The listing builds one solid part. Answer for the finished solid, in the listing's coordinates (mm). Face numbers are marked on the shaded views. A direction names the side the tool comes from. Coordinates: 2 decimals unless noted, no trailing zeros. Loops run counter-clockwise (first coordinate to the right, second up) from the corner with the lowest first, then second, coordinate; pieces in that order, holes last. Notation, with made-up numbers: (84, 29) - (138, 29) arc R17 ccw to (138, 57) - close; hole circle Ø7 at (67, 48). An arc over 180 degrees is marked (long way). Return JSON: item names as keys, results as strings. Group by question number.
1. Find the intervals of material crossed by line 1 along Y through (x, z) = (157.5, 240.5); line 2 along Z through (x, y) = (274.5, 982); line 3 along Z through (x, y) = (159, 373.5), in increasing order.
2. This flat-tipped pin is pushed along its axis until it touches: P1, Ø2, axis at x = 244.5, z = 167, coming from the -Y side. Where does it stop, or does it pass through?
3. Section C-C (y = 583.5) is taken. Write down the section's boundary in (x, z), and give its area (3 significant figures).
4. Which of the six approach directions +Z, -Z, +X, -X, +Y, -Y give full straight-line access (tool end or side, diameter ignored) to the marked faces 1 and 2?
5. Section B-B (z = 215) is taken. Write down the section's boundary in (x, y), and give its area (3 significant figures).
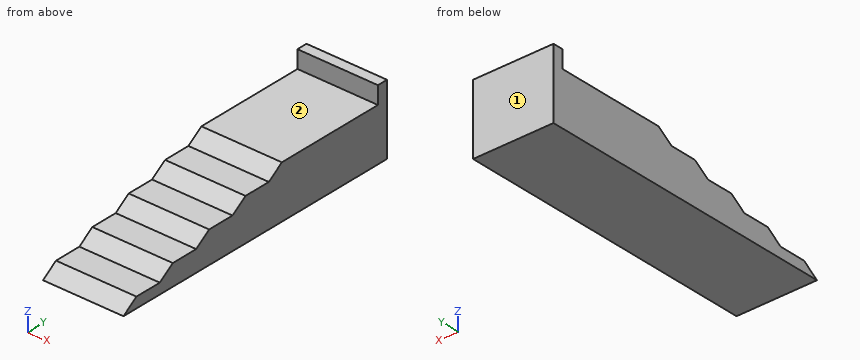
```python
from build123d import *

# Parameters (mm, degrees)
F0_W        = 1066.8
F0_H        = 38.1
F1_DEPTH    = 292.1
F2_W        = 914.4
F2_H        = 38.1
F3_DEPTH    = 292.1
F4_W        = 762
F4_H        = 38.1
F5_DEPTH    = 292.1
F6_W        = 609.6
F6_H        = 38.1
F7_DEPTH    = 292.1
F8_W        = 457.2
F8_H        = 38.1
F9_DEPTH    = 292.1
F10_SIZE2   = 54.412429
F10_SIZE    = 38.09999
F10_2_SIZE2 = 54.412429
F10_2_SIZE  = 38.09999
F10_3_SIZE2 = 54.412429
F10_3_SIZE  = 38.09999
F10_4_SIZE2 = 54.412429
F10_4_SIZE  = 38.09999
F10_5_SIZE2 = 54.412429
F10_5_SIZE  = 38.09999
F11_W       = 292.1000000001
F11_H       = 38.1
F12_DEPTH   = 254


# Not quite as in the source:
# - a fillet or chamfer is up to 0.001 mm smaller than in the source, because OpenCascade refuses the exact size


with BuildPart() as f1:
    # F0 (on Right) → F1 (new body)
    with BuildSketch(Plane.YZ):
        with Locations((533.4, 19.05)):
            Rectangle(F0_W, F0_H)
    extrude(amount=F1_DEPTH)

    # F2 (on Right) → F3 (join, through all)
    with BuildSketch(Plane.YZ):
        with Locations((609.6, 57.15)):
            Rectangle(F2_W, F2_H)
    extrude(amount=F3_DEPTH)

    # F4 (on Right) → F5 (join, through all)
    with BuildSketch(Plane.YZ):
        with Locations((685.8, 95.25)):
            Rectangle(F4_W, F4_H)
    extrude(amount=F5_DEPTH)

    # F6 (on Right) → F7 (join, through all)
    with BuildSketch(Plane.YZ):
        with Locations((762, 133.35)):
            Rectangle(F6_W, F6_H)
    extrude(amount=F7_DEPTH)

    # F8 (on Right) → F9 (join, through all)
    with BuildSketch(Plane.YZ):
        with Locations((838.2, 171.45)):
            Rectangle(F8_W, F8_H)
    extrude(amount=F9_DEPTH)

    # F10 (size 38.1 and 54.4124390569 in the source; OpenCascade refuses exactly that, so slightly less here)
    f10_edges = [f1.edges().sort_by_distance(p)[0] for p in [
        (146.05, 0, 38.1),
    ]]
    f10_side = f1.faces().sort_by_distance((146.05, 0, 19.05))[0]
    chamfer(f10_edges, length=F10_SIZE, length2=F10_SIZE2, reference=f10_side)

    # F10#2 (size 38.1 and 54.4124390569 in the source; OpenCascade refuses exactly that, so slightly less here)
    f10_2_edges = [f1.edges().sort_by_distance(p)[0] for p in [
        (146.05, 152.4, 76.2),
    ]]
    f10_2_side = f1.faces().sort_by_distance((146.05, 152.4, 57.15))[0]
    chamfer(f10_2_edges, length=F10_2_SIZE, length2=F10_2_SIZE2, reference=f10_2_side)

    # F10#3 (size 38.1 and 54.4124390569 in the source; OpenCascade refuses exactly that, so slightly less here)
    f10_3_edges = [f1.edges().sort_by_distance(p)[0] for p in [
        (146.05, 304.8, 114.3),
    ]]
    f10_3_side = f1.faces().sort_by_distance((146.05, 304.8, 95.25))[0]
    chamfer(f10_3_edges, length=F10_3_SIZE, length2=F10_3_SIZE2, reference=f10_3_side)

    # F10#4 (size 38.1 and 54.4124390569 in the source; OpenCascade refuses exactly that, so slightly less here)
    f10_4_edges = [f1.edges().sort_by_distance(p)[0] for p in [
        (146.05, 457.2, 152.4),
    ]]
    f10_4_side = f1.faces().sort_by_distance((146.05, 457.2, 133.35))[0]
    chamfer(f10_4_edges, length=F10_4_SIZE, length2=F10_4_SIZE2, reference=f10_4_side)

    # F10#5 (size 38.1 and 54.4124390569 in the source; OpenCascade refuses exactly that, so slightly less here)
    f10_5_edges = [f1.edges().sort_by_distance(p)[0] for p in [
        (146.05, 609.6, 190.5),
    ]]
    f10_5_side = f1.faces().sort_by_distance((146.05, 609.6, 171.45))[0]
    chamfer(f10_5_edges, length=F10_5_SIZE, length2=F10_5_SIZE2, reference=f10_5_side)

    # F11 (on Top) → F12 (join)
    with BuildSketch(Plane.XY):
        with Locations((146.0500000001, 1085.85)):
            Rectangle(F11_W, F11_H)
    extrude(amount=F12_DEPTH)


solid = f1.part
```
The answers:
{
 "1": {"line 1": "y = 1066.8 to 1104.9", "line 2": "z = 0 to 190.5", "line 3": "z = 0 to 114.3"},
 "2": {"P1": "stops at y = 629.02"},
 "3": {"outline": "(0, 0) - (292.1, 0) - (292.1, 152.4) - (0, 152.4) - close", "area": "44,500 mm2"},
 "4": {"face 1": "+Z, -Z, +X, -X, +Y", "face 2": "+Z, +X, -X, -Y"},
 "5": {"outline": "(0, 1066.8) - (292.1, 1066.8) - (292.1, 1104.9) - (0, 1104.9) - close", "area": "11,100 mm2"}
}
